The model under review builds one solid part; all positions refer to its coordinate system, in mm. A direction names the side the tool comes from. Round coordinates to 2 decimals unless told otherwise and drop trailing zeros. Write each loop counter-clockwise with the first axis right and the second up, starting at its lowest first coordinate (ties: lowest second). Pieces come first, ordered by that corner, then holes. Notation, with made-up numbers: (80, -27) -> (97, -27) arc R37 ccw to (97, 10) -> close; hole circle Ø4 at (-10, 10.25). An arc over 180 degrees is marked (long way). Answer as a JSON object with one key per item and string values. Group by question number.
1) Insertion check: pin 1 Ø4 at (y, z) = (10, 48.5) entering from -X; pin 2 Ø8 at (y, z) = (16.5, 34.5) entering from -X; pin 3 Ø6 at (x, y) = (26, 15) entering from +Z. Each pin has a flat end and moves straight along its axis. Give the tip position at first contact, or say it passes through.
2) We need section C-C, the plane y = 11. Write out the cut boundary in (x, z).
3) To check wall thickness, follow probe 1 along Z at (x, y) = (0, 6.5); probe 2 along X at (y, z) = (8.5, -1.5). State the ranges of each line that lie inside material, in increasing order. Write a range as [from, to].
4) Mouldability with a two-part tool opening along X and no side actions: class faces 1 (the cylindrical face through (48.43, 12.52, -15.25)), 2 (the flat face through (-35.4, 7.175, -55.5)), 3 (the cylindrical face through (-64.564, 3.537, -20.332)) as pulls with the +X half, pulls with the -X half, needs draft (parallel to the pull), parting line crosses it, or undercut.
5) Machinability: for faces 4 (the flat face through (0, 0, -51)), 5 (the flat face through (58, 2, 0)), 6 (the cylindrical face through (-57.095, 15.399, -2.513)), which of the approach directions +Z, -Z, +X, -X, +Y, -Y give a long, thin tool a straight path to every point of the face, cutting with its end or side? Answer none if there is none.
from build123d import *

# Parameters (mm, degrees)
SKETCH1_R           = 57.15
SKETCH1_R_2         = 50.7746
BOSS_EXTRUDE1_DEPTH = 25.4
FILLET1_R           = 0.5


with BuildPart() as part:
    # Sketch1 → Boss-Extrude1 (new body)
    with BuildSketch(Plane(origin=(0, 0, 0), x_dir=(1, 0, 0), z_dir=(0, 1, 0))):
        Circle(SKETCH1_R)
        Circle(SKETCH1_R_2, mode=Mode.SUBTRACT)
    extrude(amount=BOSS_EXTRUDE1_DEPTH)

    # Sketch2 → Revolve1 (revolve)
    with BuildSketch(Plane.XY):
        Polygon((-57.15, 5.175), (-65.15, 5.175), (-65.15, 7.175), (-67.69, 7.175), (-67.69, 0), (-65.15, 0), (-65.15, 2), (-57.15, 2), align=None)
    revolve(axis=Axis((0, 25.4, 0), (0, -1, 0)))

    # Fillet1
    fillet1_edges = [part.edges().sort_by_distance(p)[0] for p in [
        (-57.15, 5.175, 0),
        (-57.15, 2, 0),
        (65.15, 2, 0),
        (65.15, 5.175, 0),
    ]]
    fillet(fillet1_edges, radius=FILLET1_R)


solid = part.part
Here are the results:
{
 "1": {"pin 1": "stops at x = -33.22", "pin 2": "stops at x = -48.33", "pin 3": "stops at z = 52.32"},
 "2": {"outline": "circle Ø114.3 at (0, 0); hole circle Ø101.55 at (0, 0)"},
 "3": {"probe 1": "z = [-67.69, -65.15], [-57.15, -50.77], [50.77, 57.15], [65.15, 67.69]", "probe 2": "x = [-57.13, -50.75], [50.75, 57.13]"},
 "4": {"face 1": "undercut", "face 2": "needs draft", "face 3": "parting line crosses it"},
 "5": {"face 4": "+Z, -Z, +X, -X, -Y", "face 5": "-Y", "face 6": "+Y"}
}
